```python
from build123d import *

# Parameters (mm, degrees)
RADYUS2_R = 0.5


with BuildPart() as part:
    # Çizim1 → Döndür2 (revolve)
    with BuildSketch(Plane.XY):
        Polygon((0, 0), (0, 8), (22.5, 8), (22.5, 9), (58.5, 9), (58.5, 8), (81, 8), (81, 0), align=None)
    revolve(axis=Axis((81, 0, 0), (-1, 0, 0)))

    # Radyus2
    radyus2_edges = [part.edges().sort_by_distance(p)[0] for p in [
        (58.5, -8, 0),
        (22.5, -8, 0),
    ]]
    fillet(radyus2_edges, radius=RADYUS2_R)


solid = part.part
```
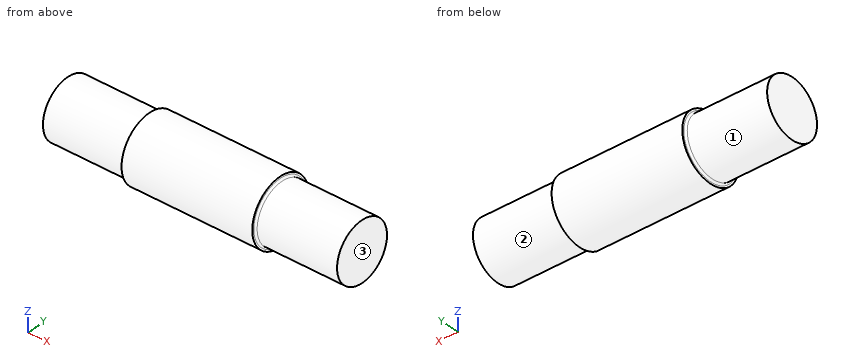
Check sheet for the modelled part. Datum: model origin and axes. Units: mm. Face numbers are marked on the shaded views. A direction names the side the tool comes from. Round coordinates to 2 decimals unless told otherwise and drop trailing zeros. Loops run counter-clockwise (first coordinate to the right, second up) from the corner with the lowest first, then second, coordinate; pieces in that order, holes last. Notation, with made-up numbers: (38.5, 45.25) -> (66.5, 45.25) arc R22 cw to (66.5, 52.25) -> close; hole circle Ø11 at (87, 54.25). An arc over 180 degrees is marked (long way). Answer in a Markdown table with one row per item.
Q1. Go/stop test with flat-tipped pins: P1, Ø3, axis at x = 54.5, z = 3, coming from the -Y side; P2, Ø4, axis at x = 70.5, z = 0.5, coming from the -Y side; P3, Ø3, axis at x = 70.5, z = -3, coming from the +Y side. Record where each tip stops, or that it passes through.
Data:
| item | result |
|---|---|
| P1 | stops at y = -8.87 |
| P2 | stops at y = -8 |
| P3 | stops at y = 7.86 |
Q2. Sectioned sample at C-C on x = 20. Enter the section's corners in (y, z).
Data:
| item | result |
|---|---|
| outline | circle Ø16 at (0, 0) |
Q3. Sectioned sample at D-D on x = 37.5. Enter the section's corners in (y, z).
Data:
| item | result |
|---|---|
| outline | circle Ø18 at (0, 0) |
Q4. Thickness scan on L1, parallel to X at y = -7.25, z = -5; L2, parallel to Y at x = 42, z = 0.25; L3, parallel to Z at x = 18.5, y = -6.5. Record the ranges inside material, lowest first.
Data:
| item | result |
|---|---|
| L1 | x = 22.5 to 58.5 |
| L2 | y = -9 to 9 |
| L3 | z = -4.66 to 4.66 |
Q5. Sectioned sample at A-A on y = 0. Enter the section's corners in (x, z), then the cut area to 3 significant figures.
Data:
| item | result |
|---|---|
| outline | (0, -8) -> (22, -8) arc R0.5 cw to (22.5, -8.5) -> (22.5, -9) -> (58.5, -9) -> (58.5, -8.5) arc R0.5 cw to (59, -8) -> (81, -8) -> (81, 8) -> (59, 8) arc R0.5 cw to (58.5, 8.5) -> (58.5, 9) -> (22.5, 9) -> (22.5, 8.5) arc R0.5 cw to (22, 8) -> (0, 8) -> close |
| area | 1,370 mm^2 |
Q6. Set-up check for the marked faces 1, 2 and 3: record each of +Z, -Z, +X, -X, +Y, -Y from which the full face is reachable in a straight line by a thin tool's end or side.
Data:
| item | result |
|---|---|
| face 1 | -X |
| face 2 | +X |
| face 3 | +Z, -Z, +X, +Y, -Y |
